Autodesk Fusion 360 part; units mm, degrees
sketch "Sketch1" plane through (0, 0, 0) normal (0, 0, 1) x (1, 0, 0)
  line L0 (-13, 8) -> (20, 8)
  line L1 (20, 8) -> (20, 3)
  line L2 (20, 3) -> (-13, 3)
  line L3 (-13, 3) -> (-13, 8)
  line L4 (-13, 8) -> (-7.8, 8)
  line L5 (-7.8, 8) -> (-7.8, 25)
  line L6 (-7.8, 25) -> (-13, 25)
  line L7 (-13, 25) -> (-13, 8)
  line L8 (20, 8) -> (14.8, 8)
  line L9 (14.8, 8) -> (14.8, 25)
  line L10 (14.8, 25) -> (20, 25)
  line L11 (20, 25) -> (20, 8)
  dimension "d1" = 33
  dimension "d2" = 5
  dimension "d3" = 5.2
  dimension "d4" = 17
  dimension "d5" = 17
  dimension "d6" = 5.2
extrude "Extrude1" add sketch "Sketch1" along normal blind 22
sketch "Sketch2" plane through (0, 0, 22) normal (0, 0, 1) x (1, 0, 0)
  line L0 (-7.8, 8) -> (-7.8, 25)
  line L1 (-7.8, 25) -> (-13, 25)
  line L2 (-13, 25) -> (-13, 3)
  line L3 (-13, 3) -> (20, 3)
  line L4 (20, 3) -> (20, 25)
  line L5 (20, 25) -> (14.8, 25)
  line L6 (14.8, 25) -> (14.8, 8)
  line L7 (14.8, 8) -> (-7.8, 8)
  line L8 (-13, 25) -> (-7.8, 25)
  line L9 (-7.8, 25) -> (-7.8, 8)
  line L10 (-7.8, 8) -> (-13, 8)
  line L11 (-13, 8) -> (-13, 25)
  line L12 (14.8, 25) -> (20, 25)
  line L13 (20, 25) -> (20, 8)
  line L14 (20, 8) -> (14.8, 8)
  line L15 (14.8, 8) -> (14.8, 25)
  line L16 (20, 25) -> (14.8, 25)
  line L17 (14.8, 25) -> (14.8, 8)
  line L18 (14.8, 8) -> (20, 8)
  line L19 (20, 8) -> (20, 25)
  line L20 (-7.8, 25) -> (-13, 25)
  line L21 (-13, 25) -> (-13, 8)
  line L22 (-13, 8) -> (-7.8, 8)
  line L23 (-7.8, 8) -> (-7.8, 25)
  point P0 (20, 8)
  dimension "d9" = 17
  dimension "d10" = 5.2
  dimension "d15" = 5.2
  dimension "d16" = 17
extrude "Extrude5" cut sketch "Sketch1" along normal blind 5 contours L0 L4 L5 L6 L7
extrude "Extrude4" cut sketch "Sketch1" along normal blind 5 contours L0 L8 L9 L10 L11
extrude "Extrude3" cut sketch "Sketch2" against normal blind 5 contours L4 L5 L6 L12 L13 L14 L15 L16 L17 L18 L19
extrude "Extrude2" cut sketch "Sketch2" against normal blind 5 contours L0 L1 L2 L8 L9 L10 L11 L20 L21 L22 L23
extrude "Extrude6" add sketch "Sketch1" against normal blind 7 contours L0 L1 L2 L3 L4 L8
extrude "Extrude7" add sketch "Sketch2" along normal blind 7 contours L2 L3 L4 L7 L10 L14 L18 L22
sketch "Sketch3" plane through (20, 0, 0) normal (1, 0, 0) x (0, 0, -1)
  line L0 (-17, 25) -> (-17, 8)
  line L1 (-17, 8) -> (-29, 8)
  line L2 (-29, 8) -> (-29, 3)
  line L3 (-29, 3) -> (7, 3)
  line L4 (7, 3) -> (7, 8)
  line L5 (7, 8) -> (-5, 8)
  line L6 (-5, 8) -> (-5, 25)
  line L7 (-5, 25) -> (-17, 25)
  line L8 (-17, 8) -> (-8, 8)
  line L9 (-8, 8) -> (-8, 16)
  line L10 (-8, 16) -> (-17, 16)
  line L11 (-17, 16) -> (-17, 8)
extrude "Extrude8" cut sketch "Sketch3" against normal blind 9 contours L0 L8 L9 L10 L11
chamfer "Chamfer1" distance 0.5 angle 45 1 edges at (17.4, 25, 17)
fillet "Fillet1" radius 0.5 1 edges at (-10.4, 25, 17)
fillet "Fillet2" radius 0.5 1 edges at (-10.4, 25, 5)
fillet "Fillet3" radius 0.5 1 edges at (17.4, 25, 5)
fillet "Fillet4" radius 0.5 2 edges at (3.5, 8, 29) (3.5, 8, -7)
sketch "Sketch4" plane through (0, 25, 0) normal (0, 1, 0) x (-1, 0, 0)
  line L0 (7.8, 5.5) -> (13, 5.5)
  line L1 (13, 5.5) -> (13, 16.5)
  line L2 (13, 16.5) -> (7.8, 16.5)
  line L3 (7.8, 16.5) -> (7.8, 5.5)
  circle A0 centre (10.4, 11) radius 1.25
  circle A1 centre (-17.4, 11) radius 1.25
  dimension "d32" = 2.5
  dimension "d33" = 2.5
extrude "Extrude9" cut sketch "Sketch4" against normal blind 5 contours A0
extrude "Extrude10" cut sketch "Sketch4" against normal blind 5 contours A1
Model file for the job. Use its own axes, mm. A direction names the side the tool comes from. Give positions to 0.01 mm unless a question says otherwise; leave off trailing zeros. Write each loop counter-clockwise with the first axis right and the second up, starting at its lowest first coordinate (ties: lowest second). Pieces come first, ordered by that corner, then holes. Notation, with made-up numbers: (-17.5, 19.5) -> (14.5, 19.5) arc R18 cw to (14.5, 50.5) -> close; hole circle Ø2 at (-31.75, 6.5). An arc over 180 degrees is marked (long way). Use CSV: the item, a comma, the result in double quotes. Start each with the question number.
1) Cut at B-B on z = 15.5. List the corners of the cut face in (x, y), plus the area to 3 significant figures.
2) Cut at C-C on x = 17.4. List the corners of the cut face in (y, z).
3) Tool access for faces 1 (the flat face through (-7.8, 16, 11)), 2 (the flat face through (17, 20, 11)), 3 (the flat face through (17, 12, 8)), 4 (the flat face through (-10, 16, 5)), 5 (the flat face through (17, 20, 17)): list every direction of +Z, -Z, +X, -X, +Y, -Y with a clear straight run to the whole face (end or side of a thin tool).
4) Cut at D-D on y = 17.75. List the corners of the cut face in (x, z), plus the area to 3 significant figures.
5) Cut at A-A on y = 10. List the corners of the cut face in (x, z).
6) Drill centre lines: L1, parallel to X at y = 17, z = 15; L2, parallel to Z at x = -10.4, y = 21.45; L3, parallel to X at y = 23.25, z = 10.5. Where is each one in solid material? Low to high.
7) Pin check, flat tips, straight feed: P1, Ø4, axis at x = -7.5, y = 16, coming from the -Z side; P2, Ø1.2, axis at x = -10.5, z = 10.5, coming from the +Y side; P3, Ø1.6, axis at x = 18.5, y = 22.5, coming from the +Z side. Stop position of each tip, or through.
8) Two-plate mould, pull along Z, no slides. Class faces 6 (the flat face through (3, 5, 29)), 7 (the flat face through (-10, 20, 11)), 8 (the flat face through (20, 11, 7)): released by +Z, released by -Z, zero draft, split by the parting line, or undercut.
Final values:
1,outline,"(-13, 3) -> (20, 3) -> (20, 8) -> (-7.8, 8) -> (-7.8, 25) -> (-13, 25) -> close; (14.8, 16) -> (20, 16) -> (20, 25) -> (14.8, 25) -> close"
1,area,"300 mm2"
2,outline,"(3, -7) -> (7.5, -7) arc R0.5 ccw to (8, -6.5) -> (8, 5) -> (24.5, 5) arc R0.5 ccw to (25, 5.5) -> (25, 9.75) -> (20, 9.75) -> (20, 12.25) -> (25, 12.25) -> (25, 16.5) -> (24.5, 17) -> (16, 17) -> (16, 8) -> (8, 8) -> (8, 28.5) arc R0.5 ccw to (7.5, 29) -> (3, 29) -> close"
3,face 1,"+Z, -Z, +Y"
3,face 2,"+Y"
3,face 3,"+Z, +X"
3,face 4,"-Z, +X, -X, +Y"
3,face 5,"+Z, +X, -X, +Y"
4,outline,"(-13, 5) -> (-7.8, 5) -> (-7.8, 17) -> (-13, 17) -> close; (14.8, 5) -> (20, 5) -> (20, 17) -> (14.8, 17) -> close"
4,area,"125 mm2"
5,outline,"(-13, 5) -> (-7.8, 5) -> (-7.8, 17) -> (-13, 17) -> close; (14.8, 5) -> (20, 5) -> (20, 8) -> (14.8, 8) -> close"
6,L1,"x = -13 to -7.8, 14.8 to 20"
6,L2,"z = 5 to 9.75, 12.25 to 17"
6,L3,"x = -13 to -11.55, -9.25 to -7.8, 14.8 to 16.25, 18.55 to 20"
7,P1,"stops at z = 5"
7,P2,"stops at y = 20"
7,P3,"stops at z = 17"
8,face 6,"released by +Z"
8,face 7,"undercut"
8,face 8,"zero draft"
